```python
from build123d import *

# Parameters (mm, degrees)
F1_DEPTH = 16
F2_DEPTH = 10


with BuildPart() as f1:
    # F0 (on Top) → F1 (new body)
    with BuildSketch(Plane.XY):
        with BuildLine():
            Line((-9, 9), (-9, 0))
            Line((-9, 0), (-9, -3))
            add(Edge.make_bspline(
                [(-9, -3), (-9, -2.5707676204), (-8.6315191286, -2.1415352408), (-8, -1.7474503993)],
                knots=[0, 0, 0, 0, 0.0715387299, 0.0715387299, 0.0715387299, 0.0715387299], degree=3))
            Line((-8, -1.7474503993), (-8, 0))
            Line((-8, 0), (-8, 1))
            Line((-8, 1), (-8, 8))
            Line((-8, 8), (-6, 8))
            Line((-6, 8), (-6, 9))
            Line((-6, 9), (-9, 9))
        make_face()
        with BuildLine():
            add(Edge.make_bspline(
                [(-9, -3), (-9, -2.5707676204), (-8.6315191286, -2.1415352408), (-8, -1.7474503993)],
                knots=[0, 0, 0, 0, 0.0715387299, 0.0715387299, 0.0715387299, 0.0715387299], degree=3))
            add(Edge.make_bspline(
                [(-8.8381918042, -3.5), (-8.9439804927, -3.3347222947), (-9, -3.1673611473), (-9, -3)],
                knots=[0.9721064754, 0.9721064754, 0.9721064754, 0.9721064754, 1, 1, 1, 1], degree=3))
            add(Edge.make_bspline(
                [(-8, -2.7474503993), (-8.3852847555, -2.9878784004), (-8.6726634562, -3.2413887449), (-8.8381918042, -3.5)],
                knots=[0.9284612701, 0.9284612701, 0.9284612701, 0.9284612701, 0.9721064754, 0.9721064754, 0.9721064754, 0.9721064754], degree=3))
            Line((-8, -2.7474503993), (-8, -1.7474503993))
        make_face()
        with BuildLine():
            add(Edge.make_bspline(
                [(-8.8381918042, -3.5), (-8.9439804927, -3.3347222947), (-9, -3.1673611473), (-9, -3)],
                knots=[0.9721064754, 0.9721064754, 0.9721064754, 0.9721064754, 1, 1, 1, 1], degree=3))
            Line((-9, -3), (-9, -4))
            add(Edge.make_bspline(
                [(-8.8381918042, -3.5), (-8.9439804927, -3.6652777053), (-9, -3.8326388527), (-9, -4)],
                knots=[0.9721064754, 0.9721064754, 0.9721064754, 0.9721064754, 1, 1, 1, 1], degree=3))
        make_face()
        with BuildLine():
            add(Edge.make_bspline(
                [(-8, -2.7474503993), (-8.3852847555, -2.9878784004), (-8.6726634562, -3.2413887449), (-8.8381918042, -3.5)],
                knots=[0.9284612701, 0.9284612701, 0.9284612701, 0.9284612701, 0.9721064754, 0.9721064754, 0.9721064754, 0.9721064754], degree=3))
            add(Edge.make_bspline(
                [(-8, -4.2525496007), (-8.3852847555, -4.0121215996), (-8.6726634562, -3.7586112551), (-8.8381918042, -3.5)],
                knots=[0.9284612701, 0.9284612701, 0.9284612701, 0.9284612701, 0.9721064754, 0.9721064754, 0.9721064754, 0.9721064754], degree=3))
            Line((-8, -4.2525496007), (-8, -2.7474503993))
        make_face()
        with BuildLine():
            add(Edge.make_bspline(
                [(-8.8381918042, -3.5), (-8.9439804927, -3.6652777053), (-9, -3.8326388527), (-9, -4)],
                knots=[0.9721064754, 0.9721064754, 0.9721064754, 0.9721064754, 1, 1, 1, 1], degree=3))
            add(Edge.make_bspline(
                [(-9, -4), (-9, -5.5), (0, -8.5), (9, -5.5), (9, -4)],
                knots=[0, 0, 0, 0, 0.25, 0.5, 0.5, 0.5, 0.5], degree=3))
            add(Edge.make_bspline(
                [(9, -4), (9, -3.8326388527), (8.9439804927, -3.6652777053), (8.8381918042, -3.5)],
                knots=[0.5, 0.5, 0.5, 0.5, 0.5278935246, 0.5278935246, 0.5278935246, 0.5278935246], degree=3))
            add(Edge.make_bspline(
                [(8.8381918042, -3.5), (8.6726634562, -3.7586112551), (8.3852847555, -4.0121215996), (8, -4.2525496007)],
                knots=[0.5278935246, 0.5278935246, 0.5278935246, 0.5278935246, 0.5715387299, 0.5715387299, 0.5715387299, 0.5715387299], degree=3))
            add(Edge.make_bspline(
                [(8, -4.2525496007), (6.4246057224, -5.2356378021), (0, -6.7643621979), (-6.4246057224, -5.2356378021), (-8, -4.2525496007)],
                knots=[0.5715387299, 0.5715387299, 0.5715387299, 0.5715387299, 0.75, 0.9284612701, 0.9284612701, 0.9284612701, 0.9284612701], degree=3))
            add(Edge.make_bspline(
                [(-8, -4.2525496007), (-8.3852847555, -4.0121215996), (-8.6726634562, -3.7586112551), (-8.8381918042, -3.5)],
                knots=[0.9284612701, 0.9284612701, 0.9284612701, 0.9284612701, 0.9721064754, 0.9721064754, 0.9721064754, 0.9721064754], degree=3))
        make_face()
        with BuildLine():
            add(Edge.make_bspline(
                [(8.8381918042, -3.5), (8.6726634562, -3.7586112551), (8.3852847555, -4.0121215996), (8, -4.2525496007)],
                knots=[0.5278935246, 0.5278935246, 0.5278935246, 0.5278935246, 0.5715387299, 0.5715387299, 0.5715387299, 0.5715387299], degree=3))
            add(Edge.make_bspline(
                [(8.8381918042, -3.5), (8.6726634562, -3.2413887449), (8.3852847555, -2.9878784004), (8, -2.7474503993)],
                knots=[0.5278935246, 0.5278935246, 0.5278935246, 0.5278935246, 0.5715387299, 0.5715387299, 0.5715387299, 0.5715387299], degree=3))
            Line((8, -2.7474503993), (8, -4.2525496007))
        make_face()
        with BuildLine():
            add(Edge.make_bspline(
                [(9, -3), (9, -3.1673611473), (8.9439804927, -3.3347222947), (8.8381918042, -3.5)],
                knots=[0.5, 0.5, 0.5, 0.5, 0.5278935246, 0.5278935246, 0.5278935246, 0.5278935246], degree=3))
            add(Edge.make_bspline(
                [(8, -1.7474503993), (8.6315191286, -2.1415352408), (9, -2.5707676204), (9, -3)],
                knots=[0.4284612701, 0.4284612701, 0.4284612701, 0.4284612701, 0.5, 0.5, 0.5, 0.5], degree=3))
            Line((8, -1.7474503993), (8, -2.7474503993))
            add(Edge.make_bspline(
                [(8.8381918042, -3.5), (8.6726634562, -3.2413887449), (8.3852847555, -2.9878784004), (8, -2.7474503993)],
                knots=[0.5278935246, 0.5278935246, 0.5278935246, 0.5278935246, 0.5715387299, 0.5715387299, 0.5715387299, 0.5715387299], degree=3))
        make_face()
        with BuildLine():
            add(Edge.make_bspline(
                [(8, -1.7474503993), (8.6315191286, -2.1415352408), (9, -2.5707676204), (9, -3)],
                knots=[0.4284612701, 0.4284612701, 0.4284612701, 0.4284612701, 0.5, 0.5, 0.5, 0.5], degree=3))
            Line((9, -3), (9, 0))
            Line((9, 0), (9, 9))
            Line((9, 9), (6, 9))
            Line((6, 9), (6, 8))
            Line((6, 8), (8, 8))
            Line((8, 8), (8, 1))
            Line((8, 1), (8, 0))
            Line((8, 0), (8, -1.7474503993))
        make_face()
        with BuildLine():
            add(Edge.make_bspline(
                [(9, -4), (9, -3.8326388527), (8.9439804927, -3.6652777053), (8.8381918042, -3.5)],
                knots=[0.5, 0.5, 0.5, 0.5, 0.5278935246, 0.5278935246, 0.5278935246, 0.5278935246], degree=3))
            Line((9, -4), (9, -3))
            add(Edge.make_bspline(
                [(9, -3), (9, -3.1673611473), (8.9439804927, -3.3347222947), (8.8381918042, -3.5)],
                knots=[0.5, 0.5, 0.5, 0.5, 0.5278935246, 0.5278935246, 0.5278935246, 0.5278935246], degree=3))
        make_face()
    extrude(amount=F1_DEPTH)

    # F0 (on Top) → F2 (join)
    with BuildSketch(Plane.XY):
        Polygon((-8, 0), (0, 0), (8, 0), (8, 1), (-8, 1), align=None)
    extrude(amount=F2_DEPTH)


solid = f1.part
```
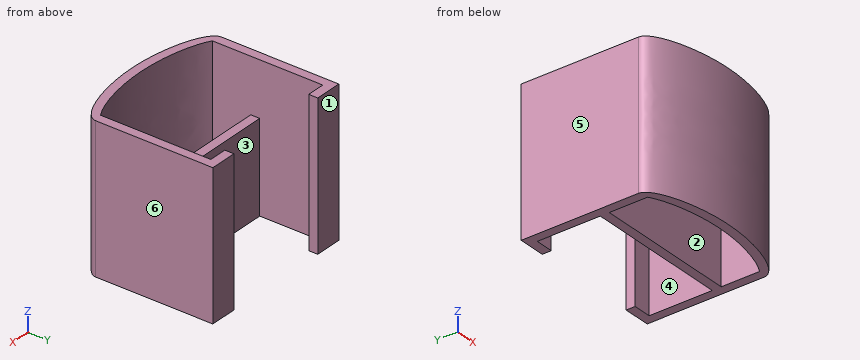
Part model, mm, in its own coordinate system. Face numbers are marked on the shaded views. A direction names the side the tool comes from. Give positions to 0.01 mm unless a question says otherwise; leave off trailing zeros. Write each loop counter-clockwise with the first axis right and the second up, starting at its lowest first coordinate (ties: lowest second). Pieces come first, ordered by that corner, then holes. Notation, with made-up numbers: (-35.75, 49) -> (16.25, 49) arc R37 cw to (16.25, 87) -> close; hole circle Ø5 at (27.25, 51). An arc over 180 degrees is marked (long way). Put each result on its own line as item: value. Start each with the question number.
Item 1: Which spindle directions (+Z, -Z, +X, -X, +Y, -Y) get a long thin tool onto all of the face, cutting with end or side? Do the marked faces 1 and 2. Say none if no direction does.
Item 2: Cut at B-B (y = 0.75). List the corners of the cut face in (x, z).
Item 3: Cut at C-C (x = -7.5). State how many separate pieces and enclosed holes the cut face has, then the cut area to 3 significant figures.
Item 4: Wall check: L1, parallel to X at y = -2.75, z = 12.5; L2, parallel to Y at x = -0.25, z = 12.75; L3, parallel to Y at x = 6.5, z = 7.25. Give the ranges that are in metal, low to high. Write a range as [from, to].
Item 5: Pull direction X, two halves, no side cores. Call the marked faces 3, 4, 5 and 6: pulls with the +X half, pulls with the -X half, needs draft (parallel to the pull), parting line crosses it, or undercut.
Item 6: Cut at A-A (y = 3.5). List the corners of the cut face in (x, z).
Item 7: Pin check, flat tips, straight feed: pin 1 Ø5 at (x, z) = (-2.5, 6.5) entering from -Y; pin 2 Ø4 at (x, y) = (-2.5, 2) entering from +Z; pin 3 Ø3 at (x, z) = (-4, 3.5) entering from +Y; pin 4 Ø0.6 at (x, z) = (-7, 11) entering from -Y. Stop position of each tip, or through.
Answer list:
1. face 1: +Z, -Z, +X, -X, +Y
1. face 2: +Z, -Z
2. outline: (-9, 0) -> (9, 0) -> (9, 16) -> (8, 16) -> (8, 10) -> (-8, 10) -> (-8, 16) -> (-9, 16) -> close
3. separate pieces: 3
3. enclosed holes: 0
3. area: 42.0 mm2
4. L1: x = [-9, -8], [8, 9]
4. L2: y = [-7, -6]
4. L3: y = [-5.95, -4.95], [0, 1], [8, 9]
5. face 3: undercut
5. face 4: undercut
5. face 5: pulls with the -X half
5. face 6: pulls with the +X half
6. outline: (-9, 0) -> (-8, 0) -> (-8, 16) -> (-9, 16) -> close; (8, 0) -> (9, 0) -> (9, 16) -> (8, 16) -> close
7. pin 1: stops at y = -7
7. pin 2: stops at z = 10
7. pin 3: stops at y = 1
7. pin 4: stops at y = -5.88
